Here's how the part is built. I have some questions about the finished solid (model axes, mm). A direction names the side the tool comes from. Round coordinates to 2 decimals unless told otherwise and drop trailing zeros. Order: outer loops, then holes, each group sorted by start corner. A loop starts at its lowest first (then second) coordinate and runs counter-clockwise, first axis right, second up. Notation, with made-up numbers: (31.5, 47.25) -> (75.5, 47.25) arc R14 ccw to (75.5, 62.25) -> close; hole circle Ø9 at (-37, 67). An arc over 180 degrees is marked (long way). Use a Markdown table: item, result. Add a question column.
(1) On a 3-axis mill with a long thin cutter (end or side, diameter ignored), from which of +Z, -Z, +X, -X, +Y, -Y can I reach the whole of each face in a straight line? I mean faces 1 (the face through (31, 9.76, 26.48)), 2 (the face through (2, 0, 67)). Say none if no direction works.
(2) I'm going to push flat-ended pins straight in: P1, Ø1, axis at x = -11, z = 31, coming from the -Y side; P2, Ø1.3, axis at x = 0.5, y = -1, coming from the +Z side; P3, Ø2.5, axis at y = 0, z = 78.5, coming from the -X side; P4, Ø4, axis at x = 6, z = 75.5, coming from the +Y side. Where does each tip first touch, or does it pass through?
(3) I want a section at B-B, the plane y = -24. Please give me the cut outline in (x, z).
(4) I want a section at D-D, the plane x = 0. Please give me the cut outline in (y, z), then the cut area to 3 significant figures.
(5) I want a section at A-A, the plane x = -24.5. Please give me the cut outline in (y, z), then the cut area to 3 significant figures.
(6) I want a section at C-C, the plane z = 26. Please give me the cut outline in (x, y).
(7) If I drill on probe 1 along X at (y, z) = (0, 69); probe 2 along Z at (x, y) = (23.5, -19); probe 3 along Y at (x, z) = (0, 75), over which ranges is the centre line in solid material (lowest first)?
(8) Thinking about a two-plate mould opening in Y: for faces 3 (the face through (-2.17, -9.76, 13.99)), 4 (the face through (14, 15, 3)), 5 (the face through (-2.5, -0.1, 70.1)), which applies, pulls with the +Y half, pulls with the -Y half, needs draft (parallel to the pull), parting line crosses it, or undercut?
from build123d import *

# Parameters (mm, degrees)
CROQUIS1_R              = 10
SALIENTE_EXTRUIR2_DEPTH = 80
CROQUIS4_R              = 32.5
SALIENTE_EXTRUIR3_DEPTH = 3
SALIENTE_EXTRUIR4_START = 25
CROQUIS5_R              = 32.5
SALIENTE_EXTRUIR4_DEPTH = 3
REDONDEO2_R             = 10
CORTAR_EXTRUIR1_START   = 80
CORTAR_EXTRUIR1_DEPTH   = 20
CORTAR_EXTRUIR2_START   = 80
CROQUIS7_W              = 3.5
CROQUIS7_H              = 7.2
CORTAR_EXTRUIR2_DEPTH   = 10
CORTAR_EXTRUIR3_START   = 1.785357468
CORTAR_EXTRUIR3_DEPTH   = 8.214642632
CORTAR_EXTRUIR4_START   = 25
CROQUIS9_R              = 2
CORTAR_EXTRUIR4_DEPTH   = 3


# Read off the part's stored shape, not the designer's step: Cortar-Extruir3
with BuildPart() as part:
    # Croquis1 → Saliente-Extruir2 (new body)
    with BuildSketch(Plane.XY):
        Circle(CROQUIS1_R)
    extrude(amount=SALIENTE_EXTRUIR2_DEPTH)

    # Croquis4 → Saliente-Extruir3 (add)
    with BuildSketch(Plane.XY):
        Circle(CROQUIS4_R)
    extrude(amount=SALIENTE_EXTRUIR3_DEPTH)

    # Croquis5 → Saliente-Extruir4 (add)
    with BuildSketch(Plane.XY.offset(SALIENTE_EXTRUIR4_START)):
        Circle(CROQUIS5_R)
    extrude(amount=SALIENTE_EXTRUIR4_DEPTH)

    # Redondeo2
    redondeo2_edges = [part.edges().sort_by_distance(p)[0] for p in [
        (-10, 0, 25),
        (-10, 0, 3),
    ]]
    fillet(redondeo2_edges, radius=REDONDEO2_R)

    # Croquis6 → Cortar-Extruir1 (cut)
    with BuildSketch(Plane.XY.offset(CORTAR_EXTRUIR1_START)):
        with BuildLine():
            Line((2, 1.5), (2, -1.5))
            ThreePointArc((2, -1.5), (-2.5, 0), (2, 1.5))
        make_face()
    extrude(amount=-CORTAR_EXTRUIR1_DEPTH, mode=Mode.SUBTRACT)

    # Croquis7 → Cortar-Extruir2 (cut)
    with BuildSketch(Plane.XY.offset(CORTAR_EXTRUIR2_START)):
        with Locations((5.5, 0)):
            Rectangle(CROQUIS7_W, CROQUIS7_H)
    extrude(amount=-CORTAR_EXTRUIR2_DEPTH, mode=Mode.SUBTRACT)

    # Cortar-Extruir3 outline → Cortar-Extruir3 (cut)
    with BuildSketch(Plane(origin=(0, 0, 0), x_dir=(0, 0, -1), z_dir=(1, 0, 0)).offset(CORTAR_EXTRUIR3_START)):
        with BuildLine():
            add(Edge.make_bspline(
                [(-73.250000008, 0), (-73.250010298, 0.457042806), (-73.439269311, 0.913556657), (-73.761440573, 1.236313288), (-74.083774062, 1.559232356), (-74.536167707, 1.749638189), (-74.998632957, 1.749999466), (-75.46109828, 1.75036072), (-75.914256207, 1.560125437), (-76.558728463, 0.916635921), (-76.75, 0.463408547), (-76.75, -0.463408547), (-76.559497121, -0.915462775), (-75.915045576, -1.559741953), (-75.458501248, -1.749734355), (-74.543528816, -1.750265056), (-74.088756627, -1.563446648), (-73.437067231, -0.912124478), (-73.250180582, -0.457964068), (-73.250000045, -0.000460382), (-73.250000003, -0.000230191), (-73.250000008, 0)],
                knots=[0.500062925, 0.500062925, 0.500062925, 0.500062925, 0.625, 0.625, 0.625000034, 0.750000005, 0.750000005, 0.750000019, 0.875000002, 0.875000002, 0.999999997, 0.999999997, 1.124999993, 1.124999993, 1.24999999, 1.24999999, 1.374999987, 1.374999987, 1.499999981, 1.499999981, 1.500062906, 1.500062906, 1.500062906, 1.500062906], degree=3))
        make_face()
    extrude(amount=CORTAR_EXTRUIR3_DEPTH, mode=Mode.SUBTRACT)

    # Croquis9 → Cortar-Extruir4 (cut)
    with BuildSketch(Plane.XY.offset(CORTAR_EXTRUIR4_START)):
        with Locations((25, 0)):
            Circle(CROQUIS9_R)
    extrude(amount=CORTAR_EXTRUIR4_DEPTH, mode=Mode.SUBTRACT)


solid = part.part
Taken from the geometry:
| question | item | result |
|---|---|---|
| 1 | face 1 | +Z, -Z |
| 1 | face 2 | +Z |
| 2 | P1 | passes through |
| 2 | P2 | stops at z = 60 |
| 2 | P3 | stops at x = -10 |
| 2 | P4 | stops at y = 9.17 |
| 3 | outline | (-21.91, 0) -> (21.91, 0) -> (21.91, 3) -> (-21.91, 3) -> close; (-21.91, 25) -> (21.91, 25) -> (21.91, 28) -> (-21.91, 28) -> close |
| 4 | outline | (-32.5, 0) -> (32.5, 0) -> (32.5, 3) -> (20, 3) arc R10 cw to (10, 13) -> (10, 15) arc R10 cw to (20, 25) -> (32.5, 25) -> (32.5, 28) -> (10, 28) -> (10, 80) -> (2.5, 80) -> (2.5, 60) -> (-2.5, 60) -> (-2.5, 80) -> (-10, 80) -> (-10, 28) -> (-32.5, 28) -> (-32.5, 25) -> (-20, 25) arc R10 cw to (-10, 15) -> (-10, 13) arc R10 cw to (-20, 3) -> (-32.5, 3) -> close |
| 4 | area | 1,860 mm2 |
| 5 | outline | (-21.35, 0) -> (21.35, 0) -> (21.35, 3) -> (-21.35, 3) -> close; (-21.35, 25) -> (21.35, 25) -> (21.35, 28) -> (-21.35, 28) -> close |
| 5 | area | 256 mm2 |
| 6 | outline | circle Ø65 at (0, 0); hole circle Ø4 at (25, 0) |
| 7 | probe 1 | x = -10 to -2.5, 2 to 10 |
| 7 | probe 2 | z = 0 to 3, 25 to 28 |
| 7 | probe 3 | y = -10 to -2.5, 2.5 to 10 |
| 8 | face 3 | parting line crosses it |
| 8 | face 4 | needs draft |
| 8 | face 5 | undercut |
